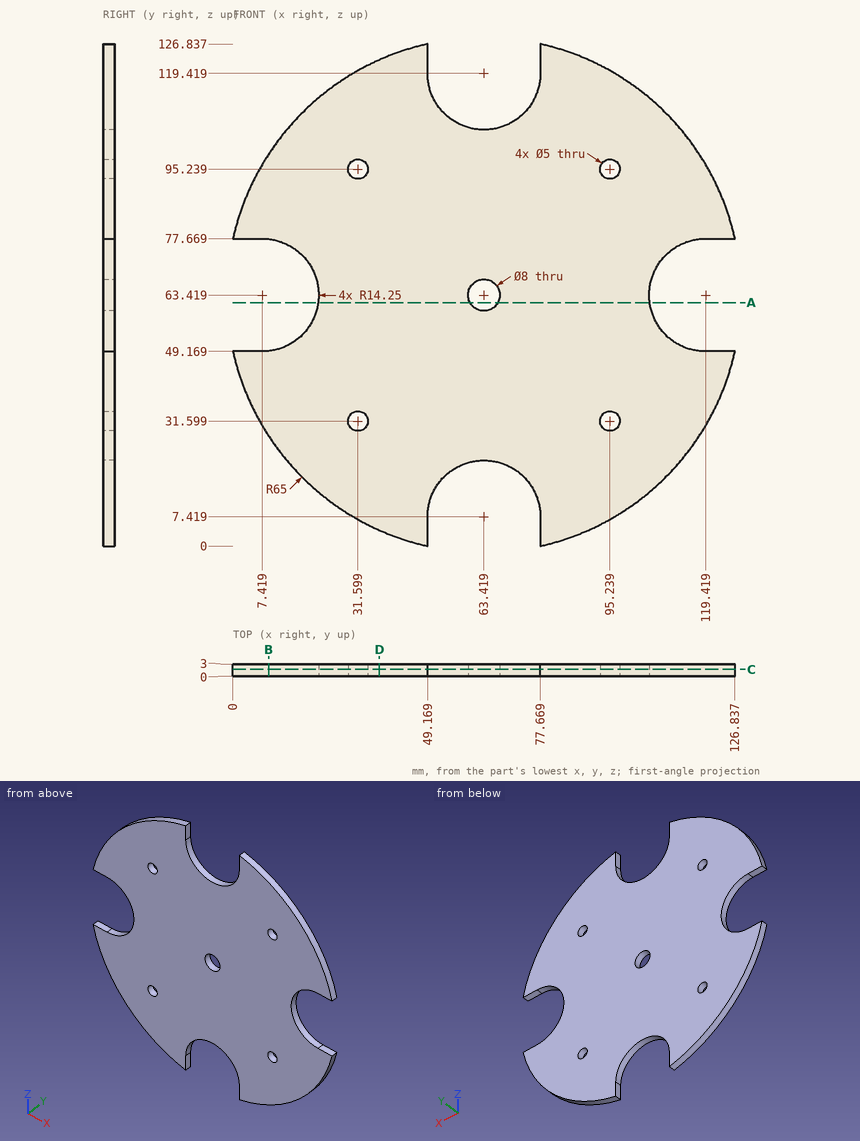
Can you work these out from the drawing? Everything is in mm from the part's minimum corner. Round coordinates to 2 decimals unless told otherwise and drop trailing zeros. Loops run counter-clockwise (first coordinate to the right, second up) from the corner with the lowest first, then second, coordinate; pieces in that order, holes last.
1. If we section it at B-B on x = 9: Write out the boundary of the cut face in (y, z) (1 decimal), plus the area to 3 significant figures.
Answer list:
outline: (0, 27.9) - (3, 27.9) - (3, 49.3) - (0, 49.3) - close; (0, 77.6) - (3, 77.6) - (3, 99) - (0, 99) - close
area: 128 mm2
2. If we section it at A-A on z = 61.5: Write out the boundary of the cut face in (x, y), plus the area to 3 significant figures.
Answer list:
outline: (21.54, 0) - (59.91, 0) - (59.91, 3) - (21.54, 3) - close; (66.93, 0) - (105.3, 0) - (105.3, 3) - (66.93, 3) - close
area: 230 mm2
3. For P1, Ø8, axis at x = 31.6, z = 95.24, coming from the +Y side; P2, Ø1.5, axis at y = 1.5, z = 121.5, coming from the -X side; P3, Ø0.9, axis at y = 1, z = 4.5, coming from the -X side (1 decimal); P4, Ø1, axis at x = 54, y = 0.5, coming from the +Z side, each with a flat end and sliding along its axis, tell me the tip position at first contact or that it passes through.
Answer list:
P1: stops at y = 3
P2: stops at x = 32.79
P3: stops at x = 35
P4: stops at z = 109.19
4. If we section it at C-C on y = 1.65: Write out the boundary of the cut face in (x, z), plus the area to 3 significant figures.
Answer list:
outline: (0, 49.17) arc R65 ccw to (49.17, 0) - (49.17, 7.42) arc R14.25 cw to (77.67, 7.42) - (77.67, 0) arc R65 ccw to (126.84, 49.17) - (119.42, 49.17) arc R14.25 cw to (119.42, 77.67) - (126.84, 77.67) arc R65 ccw to (77.67, 126.84) - (77.67, 119.42) arc R14.25 cw to (49.17, 119.42) - (49.17, 126.84) arc R65 ccw to (0, 77.67) - (7.42, 77.67) arc R14.25 cw to (7.42, 49.17) - close; hole circle Ø5 at (31.6, 31.6); hole circle Ø5 at (31.6, 95.24); hole circle Ø8 at (63.42, 63.42); hole circle Ø5 at (95.24, 31.6); hole circle Ø5 at (95.24, 95.24)
area: 10,900 mm2
5. If we section it at D-D on x = 37: Write out the boundary of the cut face in (y, z).
Answer list:
outline: (0, 4.03) - (3, 4.03) - (3, 122.81) - (0, 122.81) - close
6. If I drill on line 1 along X through (y, z) = (1.9, 63.5); line 2 along Z through (x, y) = (30.5, 2.85) (1 decimal); line 3 along X through (y, z) = (1.05, 31) (1 decimal), over which ranges is the centre line in solid material (lowest first)?
Answer list:
line 1: x = 21.67 to 59.42, 67.42 to 105.17
line 2: z = 7.4 to 29.4, 33.8 to 93, 97.5 to 119.5
line 3: x = 7.1 to 29.2, 34 to 92.8, 97.7 to 119.8
